Design review of the part built by this model. Coordinates are the model's own, in mm. A direction names the side the tool comes from. Coordinates: 2 decimals unless noted, no trailing zeros. Loops run counter-clockwise (first coordinate to the right, second up) from the corner with the lowest first, then second, coordinate; pieces in that order, holes last. Notation, with made-up numbers: M 28,21.25 L 69,21.25 A27 ccw 69,39.25 Z; hole C -5.75,-13 d8. An arc over 180 degrees is marked long. Put each result on its own line as item: value. Start each with the question number.
(1) Take a section at C-C, the plane y = -16.25. Give the boundary of the cut face in (x, z).
(2) Clearance check with flat-ended pins moving along their axes: pin 1 (5.5 mm diameter, centred on x = -0.5, z = 15.5, fed in from -Y); pin 2 (2.5 mm diameter, centred on y = -1, z = -26.5, fed in from +X); pin 3 (1.5 mm diameter, centred on x = 5, y = -15.5, fed in from +Z). State where each tip first meets the part, or that it passes through.
(3) Take a section at A-A, the plane x = 8. Give the boundary of the cut face in (y, z).
(4) Take a section at D-D, the plane z = 13. Give the boundary of the cut face in (x, y), then the cut area to 3 significant figures.
(5) For faces 5 (the flat face through (-2.5, -1, -21)), 6 (the flat face through (0, -3, 21)), 7 (the flat face through (0, 0, 9)), 8 (the flat face through (0, -1, 24.5)), 9 (the flat face through (-2.5, -1, 21)), list the 3-axis set-ups (+Z, -Z, +X, -X, +Y, -Y) from which the entire face can be reached by the end or side of a thin tool; tool diameter is ignored.
(6) The part is to be moulded in two halves that separate along Z. For faces 1 (the flat face through (1.25, -1, 27)), 2 (the flat face through (0, -1, 31.5)), 3 (the flat face through (2.5, -1, -21)), 4 (the flat face through (0, -9, 7.5)), say which applies: +Z half, -Z half, draft (parallel to the pull), parting line (faces both ways), or undercut.
(7) For probe 1 along Z at (x, y) = (6.75, -13); probe 2 along X at (y, z) = (-11.75, -7); probe 3 along Y at (x, z) = (-1.5, -17.5), list the stretches that pass through material, from the lowest coordinate up. Write a range as [from, to].
(8) Take a section at B-B, the plane y = -2.25. Give the boundary of the cut face in (x, z).
```python
from build123d import *

# Parameters (mm, degrees)
F0_W     = 5
F0_H     = 21.5
F0_W_2   = 2.5
F0_H_2   = 5
F1_DEPTH = 3
F0_H_3   = 2.5
F2_DEPTH = 18


with BuildPart() as f1:
    # F0 (on Front) → F1 (new body)
    with BuildSketch(Plane.XZ):
        with Locations((0, 20.75)):
            Rectangle(F0_W, F0_H)
        with Locations((0, 27)):
            Rectangle(F0_W_2, F0_H_2, mode=Mode.SUBTRACT)
    extrude(amount=F1_DEPTH)



with BuildPart() as f1b:
    # F0 (on Front) → F1, piece 2 (new body)
    with BuildSketch(Plane.XZ):
        with Locations((0, -20.75)):
            Rectangle(F0_W, F0_H)
        with Locations((0, -27)):
            Rectangle(F0_W_2, F0_H_2, mode=Mode.SUBTRACT)
    extrude(amount=F1_DEPTH)


with BuildPart() as f1_1:
    add(f1.part)

    add(f1b.part)  # F2 merges F1b
    # F0 (on Front) → F2 (join)
    with BuildSketch(Plane.XZ):
        with Locations((0, 8.75)):
            Rectangle(F0_W, F0_H_3)
        Polygon((10, 7.5), (10, -7.5), (2.5, -7.5), (2.5, -10), (12.5, -10), (12.5, 10), (2.5, 10), (2.5, 7.5), align=None)
        with Locations((0, -8.75)):
            Rectangle(F0_W, F0_H_3)
        Polygon((-2.5, -10), (-2.5, -7.5), (-10, -7.5), (-10, 7.5), (-2.5, 7.5), (-2.5, 10), (-12.5, 10), (-12.5, -10), align=None)
    extrude(amount=F2_DEPTH)


solid = f1_1.part
```
Computed values:
1. outline: M -12.5,-10 L 12.5,-10 L 12.5,10 L -12.5,10 Z; hole M -10,-7.5 L 10,-7.5 L 10,7.5 L -10,7.5 Z
2. pin 1: stops at y = -3
2. pin 2: stops at x = 2.5
2. pin 3: stops at z = 10
3. outline: M -18,-10 L 0,-10 L 0,-7.5 L -18,-7.5 Z; M -18,7.5 L 0,7.5 L 0,10 L -18,10 Z
4. outline: M -2.5,-3 L 2.5,-3 L 2.5,0 L -2.5,0 Z
4. area: 15.0 mm^2
5. face 5: -Z, -X, +Y, -Y
5. face 6: +Z, +X, -X, -Y
5. face 7: +Z, -Z, +X, -X, +Y
5. face 8: +Y, -Y
5. face 9: +Z, -X, +Y, -Y
6. face 1: undercut
6. face 2: +Z half
6. face 3: draft
6. face 4: undercut
7. probe 1: z = [-10, -7.5], [7.5, 10]
7. probe 2: x = [-12.5, -10], [10, 12.5]
7. probe 3: y = [-3, 0]
8. outline: M -12.5,-10 L -2.5,-10 L -2.5,-31.5 L 2.5,-31.5 L 2.5,-10 L 12.5,-10 L 12.5,10 L 2.5,10 L 2.5,31.5 L -2.5,31.5 L -2.5,10 L -12.5,10 Z; hole M -10,-7.5 L 10,-7.5 L 10,7.5 L -10,7.5 Z; hole M -1.25,-29.5 L 1.25,-29.5 L 1.25,-24.5 L -1.25,-24.5 Z; hole M -1.25,24.5 L 1.25,24.5 L 1.25,29.5 L -1.25,29.5 Z
